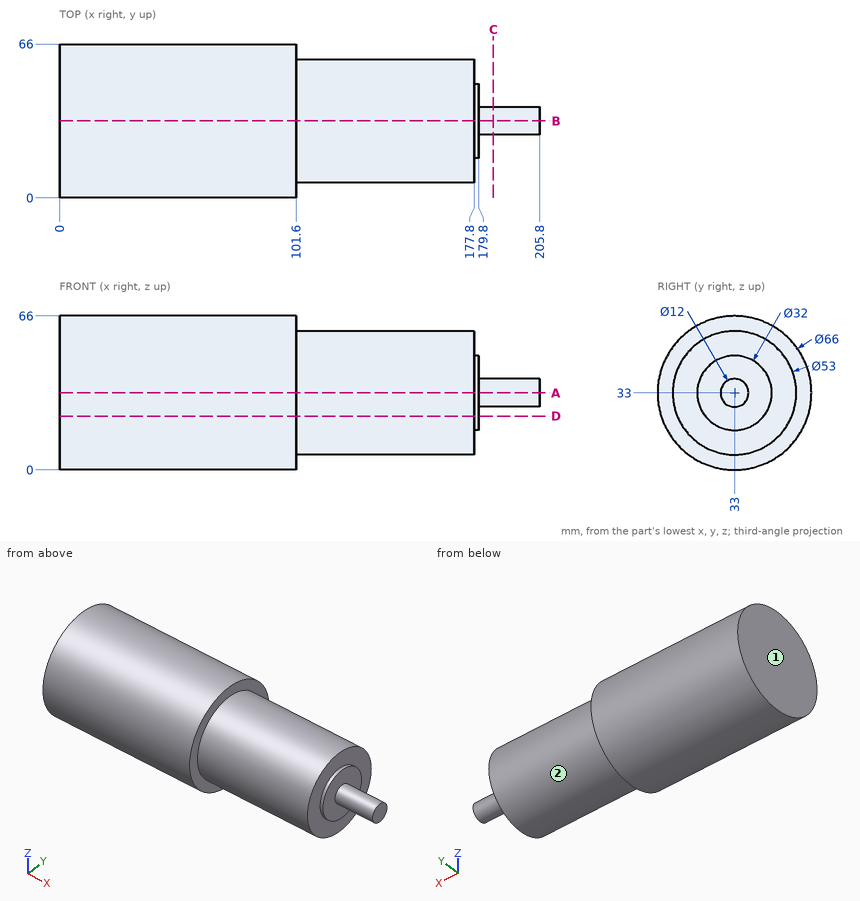
Drawing for the job (mm, zero at the part's lowest x, y, z). A direction names the side the tool comes from. Round coordinates to 2 decimals unless told otherwise and drop trailing zeros. Order: outer loops, then holes, each group sorted by start corner. A loop starts at its lowest first (then second) coordinate and runs counter-clockwise, first axis right, second up.
Item 1: Saw through at C-C on x = 186. Write the cut outline in (y, z), then the cut area to 3 significant figures.
Item 2: Saw through at D-D on z = 23. Write the cut outline in (x, y).
Item 3: Tool access for the marked faces 1 and 2: list every direction of +Z, -Z, +X, -X, +Y, -Y with a clear straight run to the whole face (end or side of a thin tool).
Item 4: Saw through at A-A on z = 33. Write the cut outline in (x, y), then the cut area to 3 significant figures.
Item 5: Probe line 1 along X through (y, z) = (23, 37); line 2 along X through (y, z) = (7.5, 42.5); line 3 along Y through (x, z) = (41, 63.5). List the from-to ranges inside material, lowest first.
Item 6: Pin check, flat tips, straight feed: pin 1 (4 mm diameter, centred on x = 72, y = 25, fed in from +Z); pin 2 (1.5 mm diameter, centred on x = 163.5, y = 30, fed in from -Z); pin 3 (6 mm diameter, centred on x = 92, y = 32.5, fed in from -Z). Stop position of each tip, or through.
Reported:
1. outline: circle Ø12 at (33, 33)
1. area: 113 mm2
2. outline: (0, 1.55) - (101.6, 1.55) - (101.6, 8.46) - (177.8, 8.46) - (177.8, 20.51) - (179.8, 20.51) - (179.8, 45.49) - (177.8, 45.49) - (177.8, 57.54) - (101.6, 57.54) - (101.6, 64.45) - (0, 64.45) - close
3. face 1: +Z, -Z, -X, +Y, -Y
3. face 2: +X
4. outline: (0, 0) - (101.6, 0) - (101.6, 6.5) - (177.8, 6.5) - (177.8, 17) - (179.8, 17) - (179.8, 27) - (205.8, 27) - (205.8, 39) - (179.8, 39) - (179.8, 49) - (177.8, 49) - (177.8, 59.5) - (101.6, 59.5) - (101.6, 66) - (0, 66) - close
4. area: 11,100 mm2
5. line 1: x = 0 to 179.8
5. line 2: x = 0 to 101.6
5. line 3: y = 20.4 to 45.6
6. pin 1: stops at z = 65.45
6. pin 2: stops at z = 6.6
6. pin 3: stops at z = 0
